Source: CAD feature listing. Evaluate the final solid. Frame: model axes, mm. A direction names the side the tool comes from. Give positions to 0.01 mm unless a question says otherwise; leave off trailing zeros. Write each loop counter-clockwise with the first axis right and the second up, starting at its lowest first coordinate (ties: lowest second). Pieces come first, ordered by that corner, then holes. Notation, with made-up numbers: (81.25, 50.25) - (97.25, 50.25) arc R13 cw to (97.25, 54.25) - close; hole circle Ø8 at (26, 12.5). An arc over 180 degrees is marked (long way). One line per question, with ' | ' between items. Start each with the question number.
(1) Draft query along Z for faces 4 (the flat face through (0, 3, -21.5)), 5 (the cylindrical face through (15.57, 2.96, -17)), 6 (the flat face through (-9, 6, 9)). Return one class per face: +Z half, -Z half, draft (parallel to the pull), parting line (faces both ways), or undercut.
(2) Section B-B, the plane z = 0. Return loops of the section in (x, y).
(3) Section A-A, the plane x = 29. Return loops of the section in (y, z).
(4) Section C-C, the plane y = -12. Return loops of the section in (x, z), plus the area to 3 significant figures.
(5) Pin query (flat end, axial travel): pin 1 (5 mm diameter, centred on y = 2, z = 6, fed in from -X); pin 2 (3 mm diameter, centred on y = 3, z = -12, fed in from +X); pin 3 (3.5 mm diameter, centred on x = -15.5, z = -15.5, fed in from -Y). Return the tip coordinate at first contact, or that it passes through.
(6) Section D-D, the plane y = -32. Return loops of the section in (x, z), plus the area to 3 significant figures.
(7) Ray query, line 1 (Y direction, x = 29, z = 19.4); line 2 (X direction, y = 3.8, z = -15.5); line 3 (Z direction, x = -15, y = 1). Return the intervals inside material, ascending. Write a range as [from, to].
(8) Access query for faces 1 (the flat face through (-21.5, 3, -3)), 2 (the flat face through (21.5, 3, -3)), 3 (the flat face through (9, 0, 9)). Directions: +Z, -Z, +X, -X, +Y, -Y. A direction counts if a zero-diameter tool reaches every point of the face in a straight line with its end or side. Return the directions, or none.
```python
from build123d import *

# Parameters (mm, degrees)
CROQUIS1_W              = 43
CROQUIS1_H              = 43
CROQUIS1_R              = 1.5
CROQUIS1_R_2            = 11.25
SALIENTE_EXTRUIR1_DEPTH = 6
CROQUIS2_W              = 15
CROQUIS2_H              = 6
SALIENTE_EXTRUIR2_DEPTH = 45
CROQUIS3_R              = 3
CORTAR_EXTRUIR1_DEPTH   = 45


with BuildPart() as part:
    # Croquis1 → Saliente-Extruir1 (new body)
    with BuildSketch(Plane(origin=(0, 0, 0), x_dir=(1, 0, 0), z_dir=(0, 1, 0))):
        Rectangle(CROQUIS1_W, CROQUIS1_H)
        with Locations(Location((-15.5, 15.5, 0), (0, 0, 270))):
            Circle(CROQUIS1_R, mode=Mode.SUBTRACT)
        with Locations(Location((15.5, 15.5, 0), (0, 0, 270))):
            Circle(CROQUIS1_R, mode=Mode.SUBTRACT)
        with Locations(Location((-15.5, -15.5, 0), (0, 0, 270))):
            Circle(CROQUIS1_R, mode=Mode.SUBTRACT)
        with Locations(Location((15.5, -15.5, 0), (0, 0, 270))):
            Circle(CROQUIS1_R, mode=Mode.SUBTRACT)
        with Locations(Location((0, 0, 0), (0, 0, 270))):
            Circle(CROQUIS1_R_2, mode=Mode.SUBTRACT)
    extrude(amount=SALIENTE_EXTRUIR1_DEPTH)

    # Croquis2 → Saliente-Extruir2 (add)
    with BuildSketch(Plane(origin=(0, 6, 0), x_dir=(1, 0, 0), z_dir=(0, 1, 0))):
        with Locations((-29, -18.5)):
            Rectangle(CROQUIS2_W, CROQUIS2_H)
        with Locations((29, -18.5)):
            Rectangle(CROQUIS2_W, CROQUIS2_H)
    extrude(amount=-SALIENTE_EXTRUIR2_DEPTH)

    # Croquis3 → Cortar-Extruir1 (cut)
    with BuildSketch(Plane(origin=(0, 0, 15.5), x_dir=(-1, 0, 0), z_dir=(0, 0, -1))):
        with Locations((-29, -32)):
            Circle(CROQUIS3_R)
        with Locations((-29, -1)):
            Circle(CROQUIS3_R)
        with Locations((29, -1)):
            Circle(CROQUIS3_R)
        with Locations((29, -32)):
            Circle(CROQUIS3_R)
    extrude(amount=-CORTAR_EXTRUIR1_DEPTH, mode=Mode.SUBTRACT)


solid = part.part
```
Check sheet entries:
1) face 4: -Z half | face 5: undercut | face 6: draft
2) outline: (-21.5, 0) - (-11.25, 0) - (-11.25, 6) - (-21.5, 6) - close; (11.25, 0) - (21.5, 0) - (21.5, 6) - (11.25, 6) - close
3) outline: (-39, 15.5) - (-35, 15.5) - (-35, 21.5) - (-39, 21.5) - close; (-29, 15.5) - (-4, 15.5) - (-4, 21.5) - (-29, 21.5) - close; (2, 15.5) - (6, 15.5) - (6, 21.5) - (2, 21.5) - close
4) outline: (-36.5, 15.5) - (-21.5, 15.5) - (-21.5, 21.5) - (-36.5, 21.5) - close; (21.5, 15.5) - (36.5, 15.5) - (36.5, 21.5) - (21.5, 21.5) - close | area: 180 mm²
5) pin 1: x = -21.5 | pin 2: x = 21.5 | pin 3: y = 0
6) outline: (-36.5, 15.5) - (-32, 15.5) - (-32, 21.5) - (-36.5, 21.5) - close; (-26, 15.5) - (-21.5, 15.5) - (-21.5, 21.5) - (-26, 21.5) - close; (21.5, 15.5) - (26, 15.5) - (26, 21.5) - (21.5, 21.5) - close; (32, 15.5) - (36.5, 15.5) - (36.5, 21.5) - (32, 21.5) - close | area: 108 mm²
7) line 1: [-39, -35], [-29, -4], [2, 6] | line 2: [-21.5, -17], [-14, 14], [17, 21.5] | line 3: [-21.5, -16.91], [-14.09, 14.09], [16.91, 21.5]
8) face 1: -Z, -X, +Y, -Y | face 2: -Z, +X, +Y, -Y | face 3: +Z, -Z, -Y
